```python
from build123d import *

# Parameters (mm, degrees)
AUFSATZ_LINEAR_AUSTRAGEN1_DEPTH      = 25
SCHNITT_LINEAR_START                 = -18
SCHNITT_LINEAR_AUSTRAGEN1_DEPTH      = 18
SCHNITT_LINEAR_AUSTRAGEN2_DEPTH      = 18
SCHNITT_LINEAR_AUSTRAGEN3_DEPTH      = 18
F_3_4_3_4_DURCHMESSER_BOHRUNG1_D     = 3.4
F_3_4_3_4_DURCHMESSER_BOHRUNG1_DEPTH = 18
F_3_0_3_DURCHMESSER_BOHRUNG2_D       = 3
FASE1_SIZE                           = 0.475
FASE1_SIZE2                          = 0.822724134
M3_GEWINDEBOHRUNG1_D                 = 2.5
M3_GEWINDEBOHRUNG1_DEPTH             = 8.5
M3_GEWINDEBOHRUNG1_TIP               = 0.751075774
F_2_5_2_5_DURCHMESSER_BOHRUNG4_D     = 2.5
F_2_5_2_5_DURCHMESSER_BOHRUNG4_DEPTH = 6
F_2_5_2_5_DURCHMESSER_BOHRUNG4_TIP   = 0.751075774
F_2_0MM_STIFTLOCH1_D                 = 2
F_2_0MM_STIFTLOCH1_DEPTH             = 8.5
F_2_0MM_STIFTLOCH1_TIP               = 0.600860619


with BuildPart() as part:
    # Skizze1 → Aufsatz-Linear austragen1 (new body)
    with BuildSketch(Plane.XY.offset(23)):
        with BuildLine():
            Line((14.492179856, 15.881647365), (6.507820144, 20.491419594))
            ThreePointArc((6.507820144, 20.491419594), (-10.75, -18.619546181), (14.492179856, 15.881647365))
        make_face()
    extrude(amount=-AUFSATZ_LINEAR_AUSTRAGEN1_DEPTH)

    # Skizze2 → Schnitt-Linear austragen1 (cut)
    with BuildSketch(Plane(origin=(0, 0, -2), x_dir=(-1, 0, 0), z_dir=(0, 0, -1)).offset(SCHNITT_LINEAR_START)):
        with BuildLine():
            Line((3.464101615, 16.4), (5.927511586, 20.66675123))
            ThreePointArc((5.927511586, 20.66675123), (0, 21.5), (-5.927511586, 20.66675123))
            Line((-5.927511586, 20.66675123), (-3.464101615, 16.4))
            ThreePointArc((-3.464101615, 16.4), (0, 14.4), (3.464101615, 16.4))
        make_face()
    extrude(amount=SCHNITT_LINEAR_AUSTRAGEN1_DEPTH, mode=Mode.SUBTRACT)

    # Skizze3 → Schnitt-Linear austragen2 (cut)
    with BuildSketch(Plane(origin=(0, 0, -2), x_dir=(-1, 0, 0), z_dir=(0, 0, -1)).offset(SCHNITT_LINEAR_START)):
        with BuildLine():
            Line((12.470765815, -11.2), (14.934175786, -15.46675123))
            ThreePointArc((14.934175786, -15.46675123), (18.619546181, -10.75), (20.861687372, -5.2))
            Line((20.861687372, -5.2), (15.93486743, -5.2))
            ThreePointArc((15.93486743, -5.2), (12.470765815, -7.2), (12.470765815, -11.2))
        make_face()
    extrude(amount=SCHNITT_LINEAR_AUSTRAGEN2_DEPTH, mode=Mode.SUBTRACT)

    # Skizze4 → Schnitt-Linear austragen3 (cut)
    with BuildSketch(Plane(origin=(0, 0, -2), x_dir=(-1, 0, 0), z_dir=(0, 0, -1)).offset(SCHNITT_LINEAR_START)):
        with BuildLine():
            Line((-15.93486743, -5.2), (-20.861687372, -5.2))
            ThreePointArc((-20.861687372, -5.2), (-18.619546181, -10.75), (-14.934175786, -15.46675123))
            Line((-14.934175786, -15.46675123), (-12.470765815, -11.2))
            ThreePointArc((-12.470765815, -11.2), (-12.470765815, -7.2), (-15.93486743, -5.2))
        make_face()
    extrude(amount=SCHNITT_LINEAR_AUSTRAGEN3_DEPTH, mode=Mode.SUBTRACT)

    # Skizze7 → Rotation1 (revolve)
    with BuildSketch(Plane.XZ, mode=Mode.PRIVATE) as rotation1_sk:
        Polygon((9.5, 34), (0, 34), (0, 23), (9.9, 23), (9.9, 31), (9.5, 31), align=None)
    revolve(rotation1_sk.sketch.rotate(Axis((0, 0, 34), (0, 0, -1)), 180), axis=Axis((0, 0, 34), (0, 0, -1)))

    # Ø3.4 (3.4) Durchmesser Bohrung1
    with Locations(Plane(origin=(0, 0, 16), x_dir=(-1, 0, 0), z_dir=(0, 0, -1))):
        with Locations((0, 18.4), (15.93486743, -9.2), (-15.93486743, -9.2)):
            Hole(F_3_4_3_4_DURCHMESSER_BOHRUNG1_D / 2, depth=F_3_4_3_4_DURCHMESSER_BOHRUNG1_DEPTH)

    # Ø3.0 (3) Durchmesser Bohrung2 (through all)
    with Locations(Plane.XY.offset(34)):
        with Locations((0, 0)):
            Hole(F_3_0_3_DURCHMESSER_BOHRUNG2_D / 2)

    # Fase1
    fase1_edges = [part.edges().sort_by_distance(p)[0] for p in [
        (1.5, 0, 34),
    ]]
    fase1_side = [part.faces().sort_by_distance(p)[0] for p in [
        (9.231299423, 0, 34),
    ]]
    chamfer(fase1_edges, length=FASE1_SIZE, length2=FASE1_SIZE2, reference=fase1_side[0])

    # M3 Gewindebohrung1
    with Locations(Plane(origin=(0, 0, -2), x_dir=(-1, 0, 0), z_dir=(0, 0, -1))):
        with Locations((-8.5, 14.722431864), (8.5, -14.722431864)):
            Hole(M3_GEWINDEBOHRUNG1_D / 2, depth=M3_GEWINDEBOHRUNG1_DEPTH)
            with Locations((0, 0, -(M3_GEWINDEBOHRUNG1_DEPTH + M3_GEWINDEBOHRUNG1_TIP / 2))):  # 118° drill point
                Cone(0, M3_GEWINDEBOHRUNG1_D / 2, M3_GEWINDEBOHRUNG1_TIP, mode=Mode.SUBTRACT)

    # Ø2.5 (2.5) Durchmesser Bohrung4
    with Locations(Plane(origin=(0, 0, -2), x_dir=(-1, 0, 0), z_dir=(0, 0, -1))):
        with Locations((-5.549084958, 9.497940228), (5.450915042, -9.554618655)):
            Hole(F_2_5_2_5_DURCHMESSER_BOHRUNG4_D / 2, depth=F_2_5_2_5_DURCHMESSER_BOHRUNG4_DEPTH)
            with Locations((0, 0, -(F_2_5_2_5_DURCHMESSER_BOHRUNG4_DEPTH + F_2_5_2_5_DURCHMESSER_BOHRUNG4_TIP / 2))):  # 118° drill point
                Cone(0, F_2_5_2_5_DURCHMESSER_BOHRUNG4_D / 2, F_2_5_2_5_DURCHMESSER_BOHRUNG4_TIP, mode=Mode.SUBTRACT)

    # Ø2.0mm Stiftloch1
    with Locations(Plane.XY.offset(23)):
        with Locations((-11.887048957, 0.988972746), (11.903074361, 0.983270441)):
            Hole(F_2_0MM_STIFTLOCH1_D / 2, depth=F_2_0MM_STIFTLOCH1_DEPTH)
            with Locations((0, 0, -(F_2_0MM_STIFTLOCH1_DEPTH + F_2_0MM_STIFTLOCH1_TIP / 2))):  # 118° drill point
                Cone(0, F_2_0MM_STIFTLOCH1_D / 2, F_2_0MM_STIFTLOCH1_TIP, mode=Mode.SUBTRACT)


solid = part.part
```
Can you work these out from the model? Positions are in its coordinate system, mm. A direction names the side the tool comes from. Coordinates: 2 decimals unless noted, no trailing zeros. Loops run counter-clockwise (first coordinate to the right, second up) from the corner with the lowest first, then second, coordinate; pieces in that order, holes last.
1) Imagine slicing it at D-D on z = 21. List the corners of the cut face in (x, y) for me, plus the area to 3 significant figures.
2) Imagine slicing it at C-C on z = 27.5. List the corners of the cut face in (x, y) for me, plus the area to 3 significant figures.
3) Which directions (+Z, -Z, +X, -X, +Y, -Y) give clear straight access to the entire face, cutting with the end or side of a thin tool? Please do faces 4 (the flat face through (-18, -5.2, 7)), 5 (the cylindrical face through (0.1, 14.4, 7.1)), 6 (the cylindrical face through (12.697, 0.375, 18.69)).
4) Imagine slicing it at B-B on y = 18.4. List the corners of the cut face in (x, z) for me, plus the area to 3 significant figures.
5) Thinking about a two-plate mould opening in X: for faces 1 (the cylindrical face through (-9.443, 2.974, 27.056)), 2 (the conical face through (-11.73, 0.92, 14)), 3 (the flat face through (13.72, -13.36, 7.13)), which applies, pulls with the +X half, pulls with the -X half, needs draft (parallel to the pull), parting line crosses it, or undercut?
6) Imagine slicing it at A-A on x = 0. List the corners of the cut face in (y, z) for me (3 decimals), plus the area to 3 significant figures.
7) I need wall thicknesses on probe 1 along Z at (x, y) = (-11.5, -16); probe 2 along Y at (x, z) = (-8.5, 3.5); probe 3 along Y at (x, z) = (4.5, 1). Which ranges of each line are inside material? Lowest first, please.
8) For pin 1 (4.5 mm diameter, centred on x = -17, y = -10, fed in from -Z); pin 2 (10 mm diameter, centred on y = 11.5, z = 22.5, fed in from -X); pin 3 (2 mm diameter, centred on y = 13.5, z = 19, fed in from -X), each with a flat end and sliding along its axis, tell me the tip position at first contact or that it passes through.
Completed:
1. outline: (6.51, 20.49) arc R21.5 ccw (long way) to (14.49, 15.88) - close; hole circle Ø3.4 at (-15.93, -9.2); hole circle Ø2 at (-11.89, 0.99); hole circle Ø3.4 at (0, 18.4); hole circle Ø3 at (0, 0); hole circle Ø2 at (11.9, 0.98); hole circle Ø3.4 at (15.93, -9.2)
1. area: 1,410 mm2
2. outline: circle Ø19.8 at (0, 0); hole circle Ø3 at (0, 0)
2. area: 301 mm2
3. face 4: -Z, -X, -Y
3. face 5: -Z, +Y
3. face 6: +Z
4. outline: (-11.12, -2) - (-4.62, -2) - (-4.62, 16) - (-1.7, 16) - (-1.7, 23) - (-11.12, 23) - close; (1.7, 16) - (4.62, 16) - (4.62, -2) - (10.13, -2) - (10.13, 23) - (1.7, 23) - close
4. area: 341 mm2
5. face 1: parting line crosses it
5. face 2: undercut
5. face 3: pulls with the +X half
6. outline: (-21.5, -2) - (-1.5, -2) - (-1.5, 33.177) - (-1.975, 34) - (-9.5, 34) - (-9.5, 31) - (-9.9, 31) - (-9.9, 23) - (-21.5, 23) - close; (1.5, -2) - (14.4, -2) - (14.4, 16) - (16.7, 16) - (16.7, 23) - (9.9, 23) - (9.9, 31) - (9.5, 31) - (9.5, 34) - (1.975, 34) - (1.5, 33.177) - close; (20.1, 16) - (21.5, 16) - (21.5, 23) - (20.1, 23) - close
6. area: 1,030 mm2
7. probe 1: z = -2 to 23
7. probe 2: y = -19.75 to -15.97, -13.47 to 19.75
7. probe 3: y = -21.02 to 8.82, 10.18 to 18.19
8. pin 1: stops at z = 16
8. pin 2: stops at x = -20.49
8. pin 3: stops at x = -17.49
